from build123d import *

# Parameters (mm, degrees)
F0_W     = 113.5
F0_H     = 113.5
F1_DEPTH = 10
F2_R     = 5
F3_R     = 4.25
F4_DEPTH = 10
F5_W     = 20
F5_H     = 51.5
F6_DEPTH = 10


with BuildPart() as f1:
    # F0 (on Top) → F1 (new body)
    with BuildSketch(Plane.XY):
        Rectangle(F0_W, F0_H)
    extrude(amount=F1_DEPTH)

    # F2
    f2_edges = [f1.edges().sort_by_distance(p)[0] for p in [
        (-56.75, -56.75, 5),
        (-56.75, 56.75, 5),
        (56.75, 56.75, 5),
        (56.75, -56.75, 5),
    ]]
    fillet(f2_edges, radius=F2_R)

    # F3 (on face) → F4 (cut)
    with BuildSketch(Plane.XY.offset(10)):
        with Locations((-44.5, -44.5)):
            Circle(F3_R)
        with Locations((44.5, -44.5)):
            Circle(F3_R)
        with Locations((-44.5, 44.5)):
            Circle(F3_R)
        with Locations((44.5, 44.5)):
            Circle(F3_R)
    extrude(amount=-F4_DEPTH, mode=Mode.SUBTRACT)

    # F5 (on face) → F6 (cut)
    with BuildSketch(Plane.XY.offset(10)):
        Rectangle(F5_W, F5_H)
    extrude(amount=-F6_DEPTH, mode=Mode.SUBTRACT)


solid = f1.part
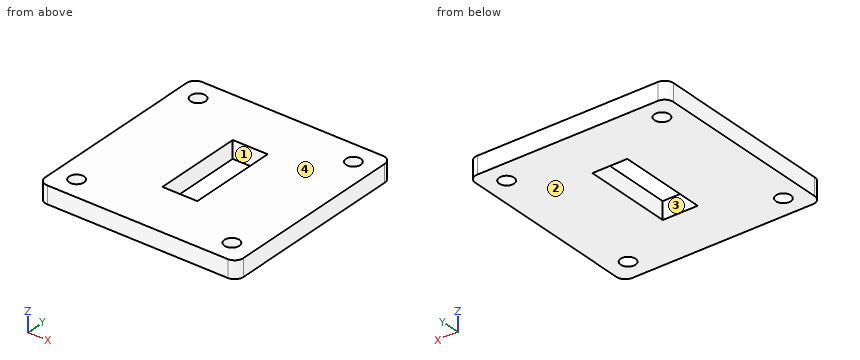
Geometry: final body of the model. Coordinates: model frame, mm. Face numbers are marked on the shaded views. A direction names the side the tool comes from. Round coordinates to 2 decimals unless told otherwise and drop trailing zeros. Order: outer loops, then holes, each group sorted by start corner. A loop starts at its lowest first (then second) coordinate and runs counter-clockwise, first axis right, second up.
Q1. Material intervals for probe 1 along Y at (x, z) = (-44.5, 4); probe 2 along Y at (x, z) = (4, 4); probe 3 along Y at (x, z) = (42, 9.25), sorted ascending.
Result sheet:
probe 1: y = -56.75 to -48.75, -40.25 to 40.25, 48.75 to 56.75
probe 2: y = -56.75 to -25.75, 25.75 to 56.75
probe 3: y = -56.75 to -47.94, -41.06 to 41.06, 47.94 to 56.75
Q2. Mould query, pull axis X, two halves, no side actions, for the marked faces 3 and 4. Classes: released by +X, released by -X, zero draft, split by the parting line, or undercut.
Result sheet:
face 3: undercut
face 4: zero draft
Q3. Section A-A, the plane x = -8. Output: boundary loops of the cut face in (y, z), and give its area (3 significant figures).
Result sheet:
outline: (-56.75, 0) - (-25.75, 0) - (-25.75, 10) - (-56.75, 10) - close; (25.75, 0) - (56.75, 0) - (56.75, 10) - (25.75, 10) - close
area: 620 mm2
Q4. Section B-B, the plane x = -44.5. Output: boundary loops of the cut face in (y, z).
Result sheet:
outline: (-56.75, 0) - (-48.75, 0) - (-48.75, 10) - (-56.75, 10) - close; (-40.25, 0) - (40.25, 0) - (40.25, 10) - (-40.25, 10) - close; (48.75, 0) - (56.75, 0) - (56.75, 10) - (48.75, 10) - close
Q5. Section C-C, the plane y = 19. Output: boundary loops of the cut face in (x, z), and give its area (3 significant figures).
Result sheet:
outline: (-56.75, 0) - (-10, 0) - (-10, 10) - (-56.75, 10) - close; (10, 0) - (56.75, 0) - (56.75, 10) - (10, 10) - close
area: 935 mm2
Q6. Access query for the marked faces 1 and 2. Directions: +Z, -Z, +X, -X, +Y, -Y. A direction counts if a zero-diameter tool reaches every point of the face in a straight line with its end or side. Return the directions, or none.
Result sheet:
face 1: +Z, -Z
face 2: -Z, +X, -X, +Y, -Y
